Geometry: final body of the model. Coordinates: model frame, mm. Face numbers are marked on the shaded views. A direction names the side the tool comes from. Give positions to 0.01 mm unless a question says otherwise; leave off trailing zeros. Write each loop counter-clockwise with the first axis right and the second up, starting at its lowest first coordinate (ties: lowest second). Pieces come first, ordered by that corner, then holes. Notation, with made-up numbers: M 57.25,88.5 L 86.25,88.5 A27 ccw 86.25,126.5 Z; hole C 81.25,-10.75 d2. An arc over 180 degrees is marked long. Use a Markdown table: item, result. Add a question column.
1) Line query: line 1 (X direction, y = 3.25, z = 6.75); line 2 (X direction, y = -3.75, z = -0.5); line 3 (Z direction, x = 27, y = -1.75). Output: solid intervals per line, ascending.
2) Section D-D on y = 6.5. Return the cut outline in (x, z), then the cut area to 3 significant figures.
3) Section C-C on x = 35. Return the cut outline in (y, z) (3 decimals).
4) Draft query along Z for the marked faces 3, 4 and 5. Return one class per face: +Z half, -Z half, draft (parallel to the pull), parting line (faces both ways), or undercut.
5) Set-up query: the marked faces 1 and 2. Return all of +Z, -Z, +X, -X, +Y, -Y with unobstructed straight access to the full face (end or side cutting, diameter ignored); none if empty.
6) Pin query (flat end, axial travel): pin 1 (6 mm diameter, centred on y = 5.5, z = 0, fed in from +X); pin 2 (10 mm diameter, centred on x = 35.5, y = 7, fed in from -Z); pin 3 (8 mm diameter, centred on x = -2, y = 1, fed in from -Z). Return the tip coordinate at first contact, or that it passes through.
```python
from build123d import *

# Parameters (mm, degrees)
SKETCH1_R           = 3.175
BOSS_EXTRUDE1_DEPTH = 57.15
CHAMFER1_SIZE       = 0.762
SKETCH6_R           = 4.7625
BOSS_EXTRUDE2_DEPTH = 6.35
SKETCH7_R           = 9.525
BOSS_EXTRUDE3_DEPTH = 6.35
CHAMFER2_SIZE       = 0.762
SKETCH8_R           = 3.175
CUT_EXTRUDE1_DEPTH  = 72.137006895
CIRPATTERN1_COUNT   = 8


with BuildPart() as part:
    # Sketch1 → Boss-Extrude1 (new body)
    with BuildSketch(Plane(origin=(0, 0, 0), x_dir=(0, 0, -1), z_dir=(1, 0, 0))):
        Circle(SKETCH1_R)
    extrude(amount=BOSS_EXTRUDE1_DEPTH)

    # Chamfer1
    chamfer1_edges = [part.edges().sort_by_distance(p)[0] for p in [
        (57.15, 0, 3.175),
    ]]
    chamfer(chamfer1_edges, length=CHAMFER1_SIZE)

    # Sketch6 → Boss-Extrude2 (add)
    with BuildSketch(Plane.ZY):
        Circle(SKETCH6_R)
    extrude(amount=BOSS_EXTRUDE2_DEPTH)

    # Sketch7 → Boss-Extrude3 (add)
    with BuildSketch(Plane.ZY.offset(6.35)):
        Circle(SKETCH7_R)
    extrude(amount=BOSS_EXTRUDE3_DEPTH)

    # Chamfer2
    chamfer2_edges = [part.edges().sort_by_distance(p)[0] for p in [
        (-6.35, 0, -9.525),
        (-12.7, 0, -9.525),
        (0, 0, -4.7625),
    ]]
    chamfer(chamfer2_edges, length=CHAMFER2_SIZE)

    # Sketch8 → Cut-Extrude1 (cut, through all)
    with BuildSketch(Plane.ZY.offset(12.7)):
        with Locations((0, 11.43)):
            Circle(SKETCH8_R)
    cut_extrude1 = extrude(amount=-CUT_EXTRUDE1_DEPTH, mode=Mode.SUBTRACT)

    # CirPattern1: Cut-Extrude1 ×8 about axis
    cirpattern1_axis = Axis((0, 0, 0), (1, 0, 0))
    for i in range(1, CIRPATTERN1_COUNT):
        add(cut_extrude1.rotate(cirpattern1_axis, i * 360 / CIRPATTERN1_COUNT), mode=Mode.SUBTRACT)


solid = part.part
```
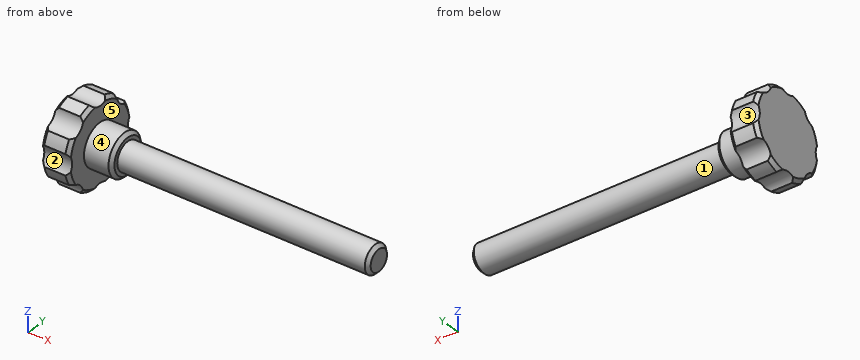
Found:
| question | item | result |
|---|---|---|
| 1 | line 1 | -12.7 to -6.35 |
| 1 | line 2 | -12.7 to 0 |
| 1 | line 3 | -2.65 to 2.65 |
| 2 | outline | M -12.7,-5.33 L -6.35,-5.33 L -6.35,5.33 L -12.7,5.33 Z |
| 2 | area | 67.7 mm² |
| 3 | outline | C 0,0 d6.35 |
| 4 | face 3 | undercut |
| 4 | face 4 | parting line |
| 4 | face 5 | draft |
| 5 | face 1 | +X |
| 5 | face 2 | +X, -X, -Y |
| 6 | pin 1 | x = 57.06 |
| 6 | pin 2 | z = -2.47 |
| 6 | pin 3 | z = -4.76 |
